Can you work these out from the model? Positions are in its coordinate system, mm. A direction names the side the tool comes from. Round coordinates to 2 decimals unless told otherwise and drop trailing zeros. Order: outer loops, then holes, each group sorted by start corner. A loop starts at its lowest first (then second) coordinate and runs counter-clockwise, first axis right, second up.
Q1. For faces 1 (the face through (31, 0, 1)), 2 (the face through (32.44, 0, 1)), 3 (the face through (-5.85, -26.36, 2.38)), which set-ups out of +Z, -Z, +X, -X, +Y, -Y let a thin tool reach every point of the face, with its end or its side?
Q2. We'd pull the mould along X, two halves only. Please class faces 4 (the face through (-29.8, 5.4, 1.2)), 5 (the face through (-32.44, 0, 1)), 6 (the face through (0, 0, 0.9)), 7 (the face through (-31.3, -0.5, 2.5)): pulls with the +X half, pulls with the -X half, needs draft (parallel to the pull), parting line crosses it, or undercut.
Q3. If we section it at B-B (x = 0): Please give me the cut outline in (y, z).
Q4. If we section it at A-A (y = 0): Please give me the cut outline in (x, z).
Q5. If we section it at C-C (z = 3.3): Please give me the cut outline in (x, y).
Q6. If we section it at D-D (y = 11.5): Please give me the cut outline in (x, z).
Q7. Will these pins go through, and if not, where does the flat tip stop? P1, Ø2, axis at x = 6.5, z = 3.5, coming from the +Y side; P2, Ø2, axis at y = -7, z = 3, coming from the -X side; P3, Ø1.5, axis at y = -18.5, z = 1, coming from the -X side.
Q8. If I drill on line 1 (X direction, y = 0, z = 1.7); line 2 (Y direction, x = 0, z = 2.4); line 3 (X direction, y = -0.5, z = 0.25), over which ranges is the centre line in solid material (lowest first)?
from build123d import *

# Parameters (mm, degrees)
PAD_DEPTH = 2.5


with BuildPart() as part:
    # Sketch → Revolution (revolve)
    with BuildSketch(Plane.XZ):
        Polygon((0, 0), (27.96, 0), (27.96, 3.9), (27, 3.9), (27, 0.9), (0, 0.9), align=None)
    revolve(axis=Axis((0, 0, 0), (0, 0, 1)))

    # Sketch001 → Pad (new body)
    with BuildSketch(Plane.XY):
        with BuildLine():
            ThreePointArc((31, 3), (29.460989, 5.620212), (26.422993, 5.552067))
            ThreePointArc((26.422993, 5.552067), (26.259684, 6.279253), (26.076366, 7.001654))
            ThreePointArc((32.44, 3), (30.363542, 6.758626), (26.076366, 7.001654))
            Line((32.44, 3), (32.44, -3))
            ThreePointArc((26.076366, -7.001654), (30.363542, -6.758626), (32.44, -3))
            ThreePointArc((26.076366, -7.001654), (26.259684, -6.279253), (26.422993, -5.552067))
            ThreePointArc((26.422993, -5.552067), (29.460989, -5.620212), (31, -3))
            Line((31, 3), (31, -3))
        make_face()
        with BuildLine():
            ThreePointArc((-26.422993, 5.552067), (-29.460989, 5.620212), (-31, 3))
            Line((-31, 3), (-31, -3))
            ThreePointArc((-31, -3), (-29.460989, -5.620212), (-26.422993, -5.552067))
            ThreePointArc((-26.422993, -5.552067), (-26.259684, -6.279253), (-26.076366, -7.001654))
            ThreePointArc((-32.44, -3), (-30.363542, -6.758626), (-26.076366, -7.001654))
            Line((-32.44, 3), (-32.44, -3))
            ThreePointArc((-26.076366, 7.001654), (-30.363542, 6.758626), (-32.44, 3))
            ThreePointArc((-26.076366, 7.001654), (-26.259684, 6.279253), (-26.422993, 5.552067))
        make_face()
    extrude(amount=PAD_DEPTH)


solid = part.part
Solution:
1. face 1: +Z, -Z
1. face 2: +Z, -Z, +X, +Y, -Y
1. face 3: +Z
2. face 4: undercut
2. face 5: pulls with the -X half
2. face 6: undercut
2. face 7: needs draft
3. outline: (-27.96, 0) - (27.96, 0) - (27.96, 3.9) - (27, 3.9) - (27, 0.9) - (-27, 0.9) - (-27, 3.9) - (-27.96, 3.9) - close
4. outline: (-32.44, 0) - (-31, 0) - (-31, 2.5) - (-32.44, 2.5) - close; (-27.96, 0) - (27.96, 0) - (27.96, 3.9) - (27, 3.9) - (27, 0.9) - (-27, 0.9) - (-27, 3.9) - (-27.96, 3.9) - close; (31, 0) - (32.44, 0) - (32.44, 2.5) - (31, 2.5) - close
5. outline: circle Ø55.92 at (0, 0); hole circle Ø54 at (0, 0)
6. outline: (-25.49, 0) - (25.49, 0) - (25.49, 3.9) - (24.43, 3.9) - (24.43, 0.9) - (-24.43, 0.9) - (-24.43, 3.9) - (-25.49, 3.9) - close
7. P1: stops at y = 27.41
7. P2: stops at x = -31.15
7. P3: stops at x = -21.6
8. line 1: x = -32.44 to -31, -27.96 to -27, 27 to 27.96, 31 to 32.44
8. line 2: y = -27.96 to -27, 27 to 27.96
8. line 3: x = -32.44 to -31, -27.96 to 27.96, 31 to 32.44
